from build123d import *

# Parameters (mm, degrees)
F0_R          = 6.25
F1_DEPTH      = 50
F1_DEPTH_BACK = 10
F0_R_2        = 7
F2_DEPTH      = 40


with BuildPart() as f1:
    # F0 (on Right) → F1 (new body, two sides)
    with BuildSketch(Plane.YZ) as f1_sk:
        Circle(F0_R)
    extrude(amount=F1_DEPTH)
    extrude(f1_sk.sketch, amount=-F1_DEPTH_BACK)

    # F0 (on Right) → F2 (join)
    with BuildSketch(Plane.YZ):
        Circle(F0_R_2)
        Circle(F0_R, mode=Mode.SUBTRACT)
    extrude(amount=F2_DEPTH)


solid = f1.part
Verification items for the finished model (mm, model axes). A direction names the side the tool comes from. Give positions to 0.01 mm unless a question says otherwise; leave off trailing zeros. Write each loop counter-clockwise with the first axis right and the second up, starting at its lowest first coordinate (ties: lowest second). Pieces come first, ordered by that corner, then holes.
(1) Gauge pin test, flat ends, axial feed: pin 1 (3 mm diameter, centred on x = 33.5, z = 2, fed in from -Y); pin 2 (5 mm diameter, centred on x = 24, z = -1, fed in from +Y); pin 3 (3 mm diameter, centred on x = 25, z = 3.5, fed in from -Y); pin 4 (4 mm diameter, centred on x = 30, z = -5.5, fed in from +Y). Record the tip position at first contact, or that the pin passes through.
(2) Cross-section at B-B (z = -4). Enter the section's corners in (x, y), plus the area to 3 significant figures.
(3) Cross-section at A-A (y = 0). Enter the section's corners in (x, z).
(4) Access from +Z, -Z, +X, -X, +Y, -Y to the whole of each face (thin tool, end or side, straight path). Record for faces 1 (the face through (50, 0, 0)), 2 (the face through (-4.93, 5.96, 1.88)), 3 (the face through (45.07, 5.96, 1.88)).
(5) Material ranges on line 1 (Z direction, x = 42, y = -5.75); line 2 (Z direction, x = 44.5, y = 0.5); line 3 (Y direction, x = 28, z = -4.25), recorded low to high.
(6) Cross-section at D-D (x = 46). Enter the section's corners in (y, z).
(7) Cross-section at C-C (x = 36). Enter the section's corners in (y, z), plus the area to 3 significant figures.
Worked out:
1. pin 1: stops at y = -6.98
1. pin 2: stops at y = 7
1. pin 3: stops at y = -6.71
1. pin 4: stops at y = 6.06
2. outline: (-10, -4.8) - (0, -4.8) - (0, -5.74) - (40, -5.74) - (40, -4.8) - (50, -4.8) - (50, 4.8) - (40, 4.8) - (40, 5.74) - (0, 5.74) - (0, 4.8) - (-10, 4.8) - close
2. area: 652 mm2
3. outline: (-10, -6.25) - (0, -6.25) - (0, -7) - (40, -7) - (40, -6.25) - (50, -6.25) - (50, 6.25) - (40, 6.25) - (40, 7) - (0, 7) - (0, 6.25) - (-10, 6.25) - close
4. face 1: +Z, -Z, +X, +Y, -Y
4. face 2: -X
4. face 3: +X
5. line 1: z = -2.45 to 2.45
5. line 2: z = -6.23 to 6.23
5. line 3: y = -5.56 to 5.56
6. outline: circle Ø12.5 at (0, 0)
7. outline: circle Ø14 at (0, 0)
7. area: 154 mm2
